Model file for the job. Use its own axes, mm. Face numbers are marked on the shaded views. Give positions to 0.01 mm unless a question says otherwise; leave off trailing zeros. Loops run counter-clockwise (first coordinate to the right, second up) from the corner with the lowest first, then second, coordinate; pieces in that order, holes last. Notation, with made-up numbers: (18, 28) - (53, 28) arc R21 ccw to (53, 46) - close; hole circle Ø8 at (79, 31.5). An arc over 180 degrees is marked (long way). Use a Markdown table: item, result.
from build123d import *

# Parameters (mm, degrees)
SKETCH_R        = 90
SKETCH_R_2      = 80
PAD_DEPTH       = 10
PAD001_DEPTH    = 10
PAD002_DEPTH    = 20
SKETCH003_W     = 8
SKETCH003_H     = 3
POCKET_DEPTH    = 26
SKETCH005_W     = 46
SKETCH005_H     = 14
POCKET001_DEPTH = 1
CHAMFER_SIZE    = 1
CHAMFER001_SIZE = 1
CHAMFER002_SIZE = 1
CHAMFER003_SIZE = 1


with BuildPart() as part:
    # Sketch → Pad (new body)
    with BuildSketch(Plane.XY):
        Circle(SKETCH_R)
        Circle(SKETCH_R_2, mode=Mode.SUBTRACT)
    extrude(amount=PAD_DEPTH)

    # Sketch001 → Pad001 (join)
    with BuildSketch(Plane.XY):
        with BuildLine():
            Line((-86.659521, -24.292538), (-140, -10))
            Line((-140, -10), (-140, 0))
            Line((-140, 0), (-90, 0))
            ThreePointArc((-90, 0), (-89.160969, -12.260569), (-86.659521, -24.292538))
        make_face()
    extrude(amount=PAD001_DEPTH)

    # Sketch002 → Pad002 (join)
    with BuildSketch(Plane.XY):
        with BuildLine():
            Line((-91, 0), (-140, 0))
            Line((-140, 0), (-140, -10))
            Line((-140, -10), (-87.780251, -23.99224))
            ThreePointArc((-91, 0), (-90.191471, -12.10366), (-87.780251, -23.99224))
        make_face()
    extrude(amount=PAD002_DEPTH)

    # Sketch003 → Pocket (cut, symmetric)
    with BuildSketch(Plane.XZ):
        with Locations((-129, 18.5)):
            Rectangle(SKETCH003_W, SKETCH003_H)
        with Locations((-99, 18.5)):
            Rectangle(SKETCH003_W, SKETCH003_H)
        with Locations((-129, 1.5)):
            Rectangle(SKETCH003_W, SKETCH003_H)
        with Locations((-99, 1.5)):
            Rectangle(SKETCH003_W, SKETCH003_H)
    extrude(amount=POCKET_DEPTH, both=True, mode=Mode.SUBTRACT)

    # Sketch005 → Pocket001 (cut, symmetric)
    with BuildSketch(Plane.XZ):
        with Locations((-117, 10)):
            Rectangle(SKETCH005_W, SKETCH005_H)
    extrude(amount=POCKET001_DEPTH, both=True, mode=Mode.SUBTRACT)

    # Chamfer
    chamfer_edges = [part.edges().sort_by_distance(p)[0] for p in [
        (-80, 0, 10),
    ]]
    chamfer(chamfer_edges, length=CHAMFER_SIZE)

    # Chamfer001
    chamfer001_edges = [part.edges().sort_by_distance(p)[0] for p in [
        (-140, -10, 15),
        (-140, -5, 20),
        (-140, 0, 18.5),
        (-140, -0.5, 17),
        (-140, -1, 13.5),
        (-140, -5.5, 10),
        (-140, -5, 0),
        (-140, 0, 1.5),
        (-140, -0.5, 3),
        (-140, -1, 6.5),
        (-140, -10, 5),
    ]]
    chamfer(chamfer001_edges, length=CHAMFER001_SIZE)

    # Chamfer002
    chamfer002_edges = [part.edges().sort_by_distance(p)[0] for p in [
        (-103, -9.95706, 20),
        (-114, -16.966679, 20),
        (-125, -7.009619, 20),
        (-114, 0, 20),
    ]]
    chamfer(chamfer002_edges, length=CHAMFER002_SIZE)

    # Chamfer003
    chamfer003_edges = [part.edges().sort_by_distance(p)[0] for p in [
        (-114, 0, 0),
        (-125, -7.009619, 0),
        (-114, -16.966679, 0),
        (-103, -9.95706, 0),
    ]]
    chamfer(chamfer003_edges, length=CHAMFER003_SIZE)


solid = part.part
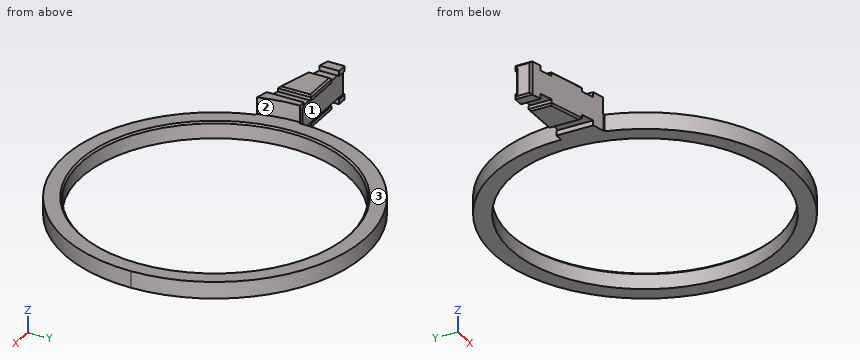
(1) Mould opens along Z. For the marked faces 1, 2 and 3 say: pulls with the +Z half, pulls with the -Z half, needs draft (parallel to the pull), parting line crosses it, or undercut.
Computed:
| item | result |
|---|---|
| face 1 | undercut |
| face 2 | needs draft |
| face 3 | pulls with the +Z half |
(2) Pin check, flat tips, straight feed: P1, Ø2, axis at x = -115.5, z = 2.5, coming from the +Y side; P2, Ø2.5, axis at y = -3.5, z = 18, coming from the +X side; P3, Ø8, axis at x = -60, z = 10, coming from the +Y side; P4, Ø6, axis at x = -85.5, y = -43, coming from the -Z side. Stop position of each tip, or through.
Computed:
| item | result |
|---|---|
| P1 | y = 0 |
| P2 | x = -90.88 |
| P3 | y = 70.46 |
| P4 | through |
(3) Slice it at A-A, the plane x = 0. Write the cut outline in (y, z).
Computed:
| item | result |
|---|---|
| outline | (-90, 0) - (-80, 0) - (-80, 9) - (-81, 10) - (-90, 10) - close; (80, 0) - (90, 0) - (90, 10) - (81, 10) - (80, 9) - close |
(4) Drill centre lines: probe 1 along Y at (x, z) = (0, 5.5); probe 2 along Z at (x, y) = (64.5, 54); probe 3 along X at (y, z) = (-55.5, 1.5). Where is each one in solid material? Low to high. Write a range as [from, to].
Computed:
| item | result |
|---|---|
| probe 1 | [-90, -80], [80, 90] |
| probe 2 | [0, 10] |
| probe 3 | [-70.85, -57.62], [57.62, 70.85] |
